For this review, use the dimensioned drawing (mm, ordinates from the lowest corner) and the shaded views. A direction names the side the tool comes from. Round coordinates to 2 decimals unless told otherwise and drop trailing zeros. Write each loop counter-clockwise with the first axis right and the second up, starting at its lowest first coordinate (ties: lowest second). Pieces come first, ordered by that corner, then holes. Notation, with made-up numbers: (17, 28.25) -> (74, 28.25) arc R28 cw to (74, 61.25) -> close; hole circle Ø8 at (-15.5, 46.5). An arc over 180 degrees is marked (long way). Answer as CSV lines item,"result". Start each with the question number.
Item 1: Machinability: for the marked faces 1 and 2, which of the approach directions +Z, -Z, +X, -X, +Y, -Y give a long, thin tool a straight path to every point of the face, cutting with its end or side? Answer none if there is none.
Item 2: Take a section at D-D on y = 21. Give the boundary of the cut face in (x, z).
Item 3: Take a section at A-A on x = 5.3. Give the boundary of the cut face in (y, z).
Item 4: Mouldability with a two-part tool opening along Z and no side actions: class the marked faces 3, 4 and 5 as +Z half, -Z half, draft (parallel to the pull), parting line (faces both ways), or undercut.
Item 5: For pin 1 Ø1.8 at (x, z) = (2, 33) entering from -Y; pin 2 Ø1.8 at (x, y) = (4, 43.5) entering from -Z, all flat-tipped, find the tip position at first contact; note any pin that passes through.
Item 6: Take a section at B-B on y = 37. Give the boundary of the cut face in (x, z).
Item 7: Take a section at C-C on z = 32. Give the boundary of the cut face in (x, y), then the cut area to 3 significant figures.
Item 8: Wall thickness on probe 1 along Z at (x, y) = (1.8, 46) (1 decimal); probe 2 along Z at (x, y) = (1.9, 46.5); probe 3 along Y at (x, z) = (1.5, 15) (1 decimal): over which ranges is each line inside the solid? List them lowest first. Write a range as from..to.
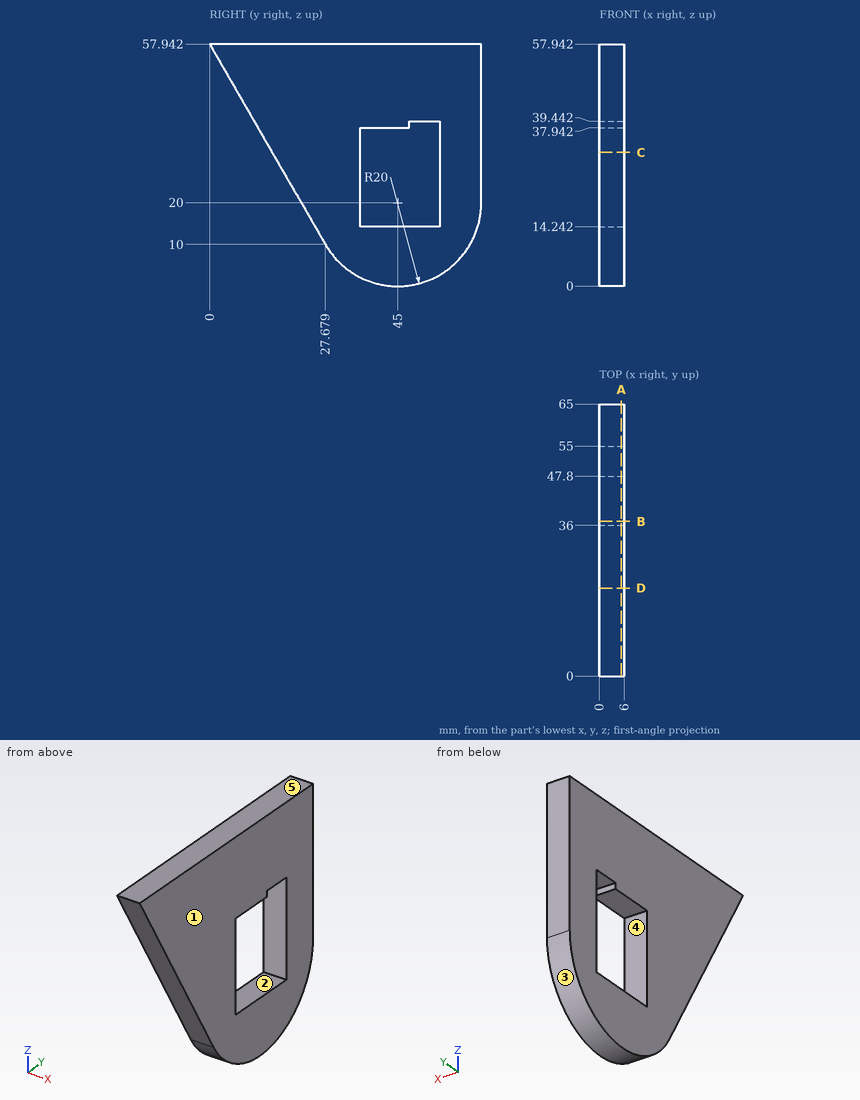
Output values:
1,face 1,"+Z, -Z, +X, +Y, -Y"
1,face 2,"+X, -X"
2,outline,"(0, 21.57) -> (6, 21.57) -> (6, 57.94) -> (0, 57.94) -> close"
3,outline,"(0, 57.94) -> (27.68, 10) arc R20 ccw to (65, 20) -> (65, 57.94) -> close; hole (36, 14.24) -> (55, 14.24) -> (55, 39.44) -> (47.8, 39.44) -> (47.8, 37.94) -> (36, 37.94) -> close"
4,face 3,"-Z half"
4,face 4,"undercut"
4,face 5,"+Z half"
5,pin 1,"stops at y = 13.88"
5,pin 2,"stops at z = 0.01"
6,outline,"(0, 1.67) -> (6, 1.67) -> (6, 14.24) -> (0, 14.24) -> close; (0, 37.94) -> (6, 37.94) -> (6, 57.94) -> (0, 57.94) -> close"
7,outline,"(0, 14.98) -> (6, 14.98) -> (6, 36) -> (0, 36) -> close; (0, 55) -> (6, 55) -> (6, 65) -> (0, 65) -> close"
7,area,"186 mm^2"
8,probe 1,"z = 0..14.2, 37.9..57.9"
8,probe 2,"z = 0.06..14.24, 37.94..57.94"
8,probe 3,"y = 24.8..36, 55..64.4"
